```python
from build123d import *

# Parameters (mm, degrees)
SCHIZZO1_W                   = 160.36
SCHIZZO1_H                   = 300
ESTRUSIONE_ESTRUSIONE1_DEPTH = 3
SCHIZZO3_R                   = 1.5
SCHIZZO3_W                   = 5
SCHIZZO3_H                   = 5
SCHIZZO3_W_2                 = 55
SCHIZZO3_H_2                 = 45
TAGLIO_ESTRUSIONE1_DEPTH     = 4
SCHIZZO4_R                   = 2
TAGLIO_ESTRUSIONE2_DEPTH     = 4
SCHIZZO5_R                   = 1.5
SCHIZZO5_W                   = 2
SCHIZZO5_H                   = 12.5
TAGLIO_ESTRUSIONE3_DEPTH     = 4
SCHIZZO6_W                   = 70
SCHIZZO6_H                   = 37
TAGLIO_ESTRUSIONE4_DEPTH     = 4


with BuildPart() as part:
    # Schizzo1 → Estrusione-Estrusione1 (new body)
    with BuildSketch(Plane(origin=(0, 0, 0), x_dir=(1, 0, 0), z_dir=(0, 1, 0))):
        Rectangle(SCHIZZO1_W, SCHIZZO1_H)
    extrude(amount=ESTRUSIONE_ESTRUSIONE1_DEPTH)

    # Schizzo3 → Taglio-Estrusione1 (cut, through all)
    with BuildSketch(Plane(origin=(0, 0, 0), x_dir=(1, 0, 0), z_dir=(0, 1, 0))):
        Circle(SCHIZZO3_R)
        with Locations((0, -100)):
            Circle(SCHIZZO3_R)
        with Locations((0, 100)):
            Circle(SCHIZZO3_R)
        with Locations((-5.042705223, -204.043249359)):
            Circle(SCHIZZO3_R)
        with Locations((-77.68, -100)):
            Rectangle(SCHIZZO3_W, SCHIZZO3_H)
        with Locations((-77.68, 0)):
            Rectangle(SCHIZZO3_W, SCHIZZO3_H)
        with Locations((-77.68, 100)):
            Rectangle(SCHIZZO3_W, SCHIZZO3_H)
        with Locations((77.68, -100)):
            Rectangle(SCHIZZO3_W, SCHIZZO3_H)
        with Locations((77.68, 0)):
            Rectangle(SCHIZZO3_W, SCHIZZO3_H)
        with Locations((77.68, 100)):
            Rectangle(SCHIZZO3_W, SCHIZZO3_H)
        with Locations((-52.68, -41.8)):
            Rectangle(SCHIZZO3_W_2, SCHIZZO3_H_2)
        with Locations((52.68, -41.8)):
            Rectangle(SCHIZZO3_W_2, SCHIZZO3_H_2)
    extrude(amount=TAGLIO_ESTRUSIONE1_DEPTH, mode=Mode.SUBTRACT)

    # Schizzo4 → Taglio-Estrusione2 (cut, through all)
    with BuildSketch(Plane(origin=(0, 0, 0), x_dir=(1, 0, 0), z_dir=(0, 1, 0))):
        with Locations((-60.18, -125)):
            Circle(SCHIZZO4_R)
        with Locations((60.18, -125)):
            Circle(SCHIZZO4_R)
        with Locations((-60.18, 125)):
            Circle(SCHIZZO4_R)
        with Locations((60.18, 125)):
            Circle(SCHIZZO4_R)
    extrude(amount=TAGLIO_ESTRUSIONE2_DEPTH, mode=Mode.SUBTRACT)

    # Schizzo5 → Taglio-Estrusione3 (cut, through all)
    with BuildSketch(Plane(origin=(0, 0, 0), x_dir=(1, 0, 0), z_dir=(0, 1, 0))):
        with Locations((72.68, 65.35)):
            Circle(SCHIZZO5_R)
        with Locations((-72.68, 65.35)):
            Circle(SCHIZZO5_R)
        with Locations((72.68, -125)):
            Circle(SCHIZZO5_R)
        with Locations((-72.68, -125)):
            Circle(SCHIZZO5_R)
        with Locations((72.68, 79.1)):
            Rectangle(SCHIZZO5_W, SCHIZZO5_H)
        with Locations((72.68, 51.6)):
            Rectangle(SCHIZZO5_W, SCHIZZO5_H)
        with Locations((-72.68, 51.6)):
            Rectangle(SCHIZZO5_W, SCHIZZO5_H)
        with Locations((-72.68, 79.1)):
            Rectangle(SCHIZZO5_W, SCHIZZO5_H)
        with Locations((72.68, -111.25)):
            Rectangle(SCHIZZO5_W, SCHIZZO5_H)
        with Locations((72.68, -138.75)):
            Rectangle(SCHIZZO5_W, SCHIZZO5_H)
        with Locations((-72.68, -111.25)):
            Rectangle(SCHIZZO5_W, SCHIZZO5_H)
        with Locations((-72.68, -138.75)):
            Rectangle(SCHIZZO5_W, SCHIZZO5_H)
    extrude(amount=TAGLIO_ESTRUSIONE3_DEPTH, mode=Mode.SUBTRACT)

    # Schizzo6 → Taglio-Estrusione4 (cut, through all)
    with BuildSketch(Plane(origin=(0, 0, 0), x_dir=(1, 0, 0), z_dir=(0, 1, 0))):
        with Locations((0, -121.5)):
            Rectangle(SCHIZZO6_W, SCHIZZO6_H)
    extrude(amount=TAGLIO_ESTRUSIONE4_DEPTH, mode=Mode.SUBTRACT)


solid = part.part
```
Work out the finished part from the listing and answer in its coordinate system (mm). Round coordinates to 2 decimals unless told otherwise and drop trailing zeros. Write each loop counter-clockwise with the first axis right and the second up, starting at its lowest first coordinate (ties: lowest second). Pieces come first, ordered by that corner, then holes. Notation, with made-up numbers: (0, 35.25) -> (37, 35.25) arc R16 ccw to (37, 58.25) -> close; hole circle Ø2 at (31, 70.25). An arc over 180 degrees is marked (long way). Write each question's results on one line, items separated by ' | '.
Q1. Flat-ended cylindrical pins translate along their axes: P1, Ø1.5, axis at y = 0.5, z = 50.5, coming from the -X side; P2, Ø0.9, axis at y = 1, z = 37.5, coming from the +X side; P3, Ø1.5, axis at y = 2, z = -1, coming from the +X side. Find the tip coordinate at first contact, or state that the pin passes through.
Data:
P1: x = -25.18 | P2: x = 25.18 | P3: x = 75.18
Q2. Straight lines are drawn through the part: line 1 along Z through (x, y) = (-27, 2.7); line 2 along Z through (x, y) = (60.18, 0.95); line 3 along Z through (x, y) = (0, 2.1). For each, find the intervals that lie inside material, in ascending order. Write a range as [from, to].
Data:
line 1: [-150, 19.3], [64.3, 103], [140, 150] | line 2: [-150, -127], [-123, 19.3], [64.3, 123], [127, 150] | line 3: [-150, -101.5], [-98.5, -1.5], [1.5, 98.5], [101.5, 103], [140, 150]
Q3. Section B-B, the plane z = 33 is taken. Write down the section's boundary in (x, y), then the cut area to 3 significant figures.
Data:
outline: (-25.18, 0) -> (25.18, 0) -> (25.18, 3) -> (-25.18, 3) -> close | area: 151 mm^2
Q4. Section A-A, the plane y = 1 is taken. Give the number of separate pieces and of enclosed holes in the cut face, then the cut area to 3 significant figures.
Data:
separate pieces: 1 | enclosed holes: 20 | area: 40,100 mm^2
